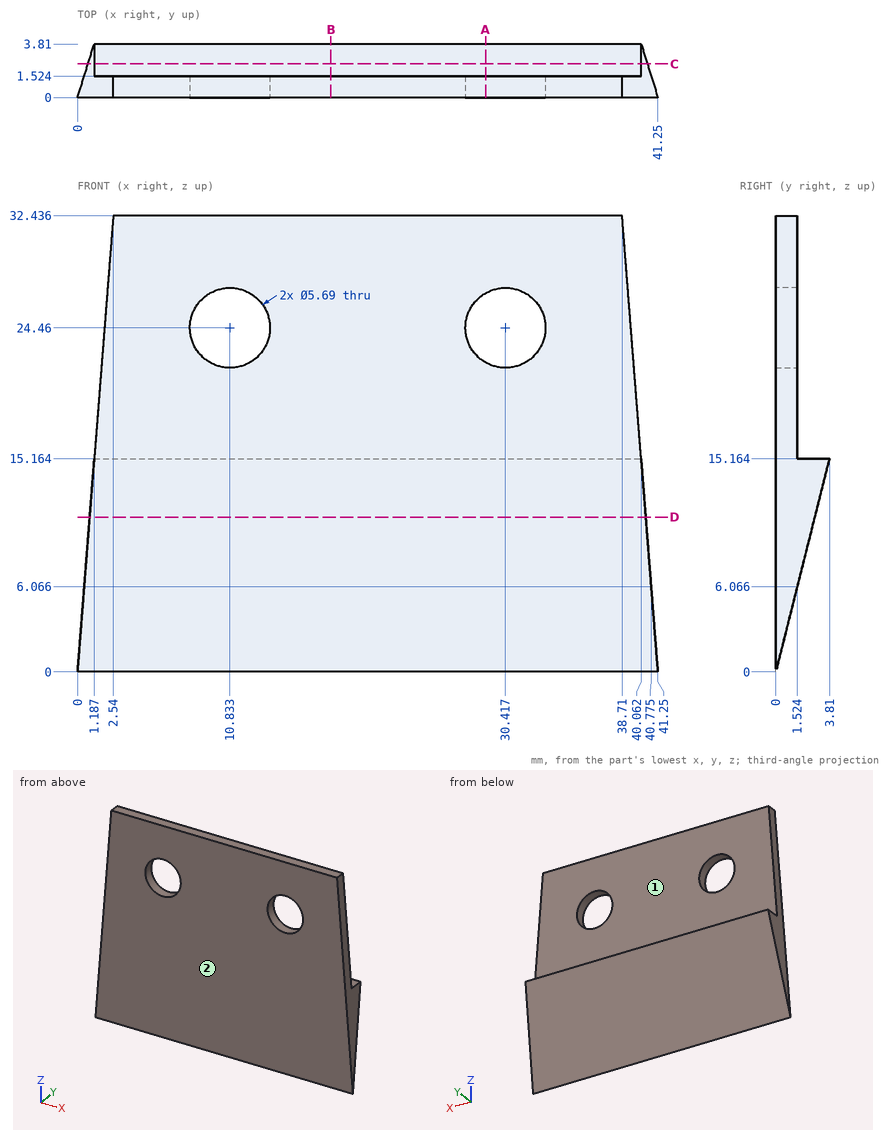
Geometry: see drawing. Coordinates: mm, zero at the bounding-box minimum. A direction names the side the tool comes from. Give positions to 0.01 mm unless a question says otherwise; leave off trailing zeros. Loops run counter-clockwise (first coordinate to the right, second up) from the corner with the lowest first, then second, coordinate; pieces in that order, holes last. Notation, with made-up numbers: M 82,8 L 109,8 A22 cw 109,20 Z; hole C 48,29 d8. An arc over 180 degrees is marked long. Answer as CSV lines item,"result". Start each with the question number.
1. Reachability of the marked faces 1 and 2 from +Z, -Z, +X, -X, +Y, -Y: full face, straight path, thin tool, end or side. Return the list, or none.
2. Pin query (flat end, axial travel): P1, Ø12, axis at x = 16.5, z = 8.5, coming from the +Y side; P2, Ø9, axis at x = 30.42, z = 24.46, coming from the -Y side; P3, Ø1.1, axis at x = 19.5, y = 3, coming from the +Z side; P4, Ø6, axis at x = 9, z = 25.5, coming from the +Y side. Return the tip coordinate at first contact, or that it passes through.
3. Section B-B on x = 18. Return loops of the section in (y, z) (1 decimal).
4. Section D-D on z = 11. Return loops of the section in (x, y).
5. Section C-C on y = 2.4. Return loops of the section in (x, z).
6. Section A-A on x = 29. Return loops of the section in (y, z) (1 decimal).
7. Line query: L1, parallel to Y at x = 15, z = 20 (1 decimal); L2, parallel to Y at x = 12, z = 10.5; L3, parallel to X at y = 0.55, z = 6. Output: solid intervals per line, ascending.
Computed values:
1,face 1,"+Z, +X, -X, +Y"
1,face 2,"+Z, -Z, +X, -X, -Y"
2,P1,"stops at y = 3.64"
2,P2,"stops at y = 0"
2,P3,"stops at z = 15.16"
2,P4,"stops at y = 1.52"
3,outline,"M 0,0 L 3.8,15.2 L 1.5,15.2 L 1.5,32.4 L 0,32.4 Z"
4,outline,"M 0.86,0 L 40.39,0 L 40.39,2.76 L 0.86,2.76 Z"
5,outline,"M 0.75,9.55 L 40.5,9.55 L 40.06,15.16 L 1.19,15.16 Z"
6,outline,"M 0,0 L 3.8,15.2 L 1.5,15.2 L 1.5,22 L 0,22 Z; M 0,26.9 L 1.5,26.9 L 1.5,32.4 L 0,32.4 Z"
7,L1,"y = 0 to 1.5"
7,L2,"y = 0 to 2.64"
7,L3,"x = 0.47 to 40.78"
